Autodesk Inventor part; units mm, degrees
ref_plane "Work Plane2" through (12.7, 0, 0) normal (1, 0, 0) x (0, 1, 0)
ref_plane "XZ Plane" through (0, 0, 0) normal (0, 1, 0) x (-1, 0, 0)
ref_plane "XY Plane" through (0, 0, 0) normal (0, 0, 1) x (1, 0, 0)
sketch "Sketch1" plane through (0, 0, 0) normal (0, 1, 0) x (-1, 0, 0)
  circle A0 centre (0, 0) radius 3.175
  circle A1 centre (0, 0) radius 3.048
  dimension "d0" = 6.35
  dimension "d1" = 6.096
extrude "Extrusion1" add sketch "Sketch1" along normal blind 127
sketch "Sketch8" plane through (0, 127, 0) normal (0, 1, 0) x (1, 0, 0)
  circle A0 centre (0, 0) radius 3.175
  circle A1 centre (0, 0) radius 3.048
extrude "Extrusion2" add sketch "Sketch8" along normal blind 7.62
sketch "Sketch16" plane through (0, 134.62, 0) normal (0, 1, 0) x (1, 0, 0)
  circle A0 centre (0, 0) radius 3.175
  circle A1 centre (0, 0) radius 3.048
extrude "Extrusion3" add sketch "Sketch16" along normal blind 17.78
sketch "Sketch17" plane through (0, 152.4, 0) normal (0, 1, 0) x (1, 0, 0)
  circle A0 centre (0, 0) radius 3.175
extrude "Extrusion4" add sketch "Sketch17" against normal blind 0.254
ref_plane "Work Plane2" through (12.7, 0, 0) normal (1, 0, 0) x (0, 1, 0)
sketch "Sketch18" plane through (12.7, 0, 0) normal (1, 0, 0) x (0, 1, 0)
  circle A0 centre (147.122, 0) radius 3.175
  point P0 (0, 0)
  dimension "d58" = 6.35
extrude "Extrusion5" cut sketch "Sketch18" against normal blind 12.7
sketch "Sketch19" plane through (0, 0, 0) normal (1, 0, 0) x (0, 0, -1)
  arc A0 (-3.175, 147.122) -> (3.175, 147.122) centre (0, 147.122) ccw
  circle A1 centre (0, 147.122) radius 3.175
  circle A2 centre (0, 147.122) radius 3.048
  point P0 (0, 0)
  dimension "d61" = 6.096
extrude "Extrusion6" add sketch "Sketch19" along normal blind 3.81
properties part number "waterpip2e"
The model under review builds one solid part; all positions refer to its coordinate system, in mm. Coordinates: 2 decimals unless noted, no trailing zeros. Loops run counter-clockwise (first coordinate to the right, second up) from the corner with the lowest first, then second, coordinate; pieces in that order, holes last. Notation, with made-up numbers: (6.25, 26.25) -> (38.25, 26.25) arc R23 cw to (38.25, 63.25) -> close; hole circle Ø5 at (82, 15.5). An arc over 180 degrees is marked (long way). Use a Markdown table: item, result. Add a question column.
1. Clearance check with flat-ended pins moving along their axes: pin 1 Ø1.5 at (y, z) = (77, -1) entering from -X; pin 2 Ø2 at (x, y) = (2.5, 136) entering from +Z; pin 3 Ø1 at (y, z) = (145, -1.5) entering from -X. State where each tip first meets the part, or that it passes through.
2. Add section B-B on y = 52.5. Write out the cut boundary in (x, z) (3 decimals), plus the area to 3 significant figures.
3. Add section A-A on z = -1. Write out the cut boundary in (x, y), plus the area to 3 significant figures.
4. To check wall thickness, follow line 1 (Y direction, x = -1.5, z = 2); line 2 (Y direction, x = 1, z = 2); line 3 (Z direction, x = -2.25, y = 41). State the ranges of each line that lie inside material, in increasing order.
Returned:
| question | item | result |
|---|---|---|
| 1 | pin 1 | stops at x = -3.17 |
| 1 | pin 2 | stops at z = 2.8 |
| 1 | pin 3 | stops at x = -3.01 |
| 2 | outline | circle Ø6.35 at (0, 0); hole circle Ø6.096 at (0, 0) |
| 2 | area | 2.48 mm² |
| 3 | outline | (-3.01, 0) -> (-2.88, 0) -> (-2.88, 152.15) -> (2.88, 152.15) -> (2.88, 150.14) -> (0, 150.14) -> (0, 150) -> (3.81, 150) -> (3.81, 150.14) -> (3.01, 150.14) -> (3.01, 152.4) -> (-3.01, 152.4) -> close; (0, 144.11) -> (2.88, 144.11) -> (2.88, 0) -> (3.01, 0) -> (3.01, 144.11) -> (3.81, 144.11) -> (3.81, 144.24) -> (0, 144.24) -> close |
| 3 | area | 42.6 mm² |
| 4 | line 1 | y = 152.15 to 152.4 |
| 4 | line 2 | y = 144.66 to 144.82, 149.42 to 149.59, 152.15 to 152.4 |
| 4 | line 3 | z = -2.24 to -2.06, 2.06 to 2.24 |
